Build history of the part. All positions in model axes, mm. A direction names the side the tool comes from. Round coordinates to 2 decimals unless told otherwise and drop trailing zeros. Write each loop counter-clockwise with the first axis right and the second up, starting at its lowest first coordinate (ties: lowest second). Pieces come first, ordered by that corner, then holes. Notation, with made-up numbers: (-39, 34) - (8, 34) arc R12 cw to (8, 41) - close; hole circle Ø3 at (64.25, -12). An arc over 180 degrees is marked (long way). Answer as a JSON object with one key per item and string values. Group by question number.
Item 1: Slice it at C-C, the plane z = -91. List the corners of the cut face in (x, y), then the cut area to 3 significant figures.
Item 2: Slice it at D-D, the plane x = 71. List the corners of the cut face in (y, z), then the cut area to 3 significant figures.
Item 3: Slice it at B-B, the plane y = 1.2. Give the number of separate pieces and of enclosed holes in the cut face, then the cut area to 3 significant figures.
Item 4: Which spindle directions (+Z, -Z, +X, -X, +Y, -Y) get a long thin tool onto all of the face, cutting with end or side? Do faces 4 (the cylindrical face through (-122.15, 2.46, 51.99)), 5 (the cylindrical face through (-112.97, 1.48, 47.21)). Say none if no direction does.
Item 5: Two-plate mould, pull along Z, no slides. Class faces 1 (the flat face through (43.7, 3, -46.3)), 2 (the flat face through (-30, 5, -30)), 3 (the cylindrical face through (57.85, 2.46, -58.01)): +Z half, -Z half, draft (parallel to the pull), parting line (faces both ways), or undercut.
Item 6: Flat gauge pins, fed straight in: pin 1 (6.5 mm diameter, centred on x = -113.5, z = 45, fed in from -Y); pin 2 (3 mm diameter, centred on y = 2.5, z = 99.5, fed in from -X); pin 3 (5 mm diameter, centred on x = 45, z = 45, fed in from -Y); pin 4 (3 mm diameter, centred on x = -115, z = -45, fed in from -Y). Where does each tip first touch, or does it go through?
Item 7: Slice it at A-A, the plane z = 20. List the corners of the cut face in (x, y).
Item 8: Probe line 1 (X direction, y = 3.5, z = -115); line 2 (X direction, y = 3.4, z = -45); line 3 (X direction, y = 4.45, z = -70.5). List the from-to ranges inside material, lowest first. Write a range as from..to.
from build123d import *

# Parameters (mm, degrees)
SKETCH_1_W          = 250
SKETCH_1_H          = 250
SKETCH_1_R          = 40
SKETCH_1_R_2        = 2.05
EXTRUDE_1_DEPTH     = 5
SKETCH_2_R          = 1.6
SKETCH_2_W          = 70
SKETCH_2_H          = 70
CUT_EXTRUDE_1_DEPTH = 177.847391838
FILLET_1_R          = 10
SKETCH_4_R          = 3
CUT_EXTRUDE_3_DEPTH = 3


with BuildPart() as part:
    # ｽｹｯﾁ1 → ﾎﾞｽ - 押し出し1 (new body)
    with BuildSketch(Plane(origin=(0, 0, 0), x_dir=(1, 0, 0), z_dir=(0, 1, 0))):
        Rectangle(SKETCH_1_W, SKETCH_1_H)
        with Locations(Location((0, 0, 0), (0, 0, 270))):
            Circle(SKETCH_1_R, mode=Mode.SUBTRACT)
        with Locations(Location((0, 60, 0), (0, 0, 270))):
            Circle(SKETCH_1_R_2, mode=Mode.SUBTRACT)
        with Locations(Location((60, 0, 0), (0, 0, 270))):
            Circle(SKETCH_1_R_2, mode=Mode.SUBTRACT)
        with Locations(Location((0, -60, 0), (0, 0, 270))):
            Circle(SKETCH_1_R_2, mode=Mode.SUBTRACT)
        with Locations(Location((-60, 0, 0), (0, 0, 270))):
            Circle(SKETCH_1_R_2, mode=Mode.SUBTRACT)
    extrude(amount=EXTRUDE_1_DEPTH)

    # ｽｹｯﾁ2 → ｶｯﾄ - 押し出し1 (cut, through all)
    with BuildSketch(Plane(origin=(0, 5, 0), x_dir=(1, 0, 0), z_dir=(0, 1, 0))):
        with Locations(Location((-45, 115, 0), (0, 0, 270))):
            Circle(SKETCH_2_R)
        with Locations(Location((-45, 45, 0), (0, 0, 270))):
            Circle(SKETCH_2_R)
        with Locations(Location((-115, 45, 0), (0, 0, 270))):
            Circle(SKETCH_2_R)
        with Locations(Location((115, 45, 0), (0, 0, 90))):
            Circle(SKETCH_2_R)
        with Locations(Location((45, 115, 0), (0, 0, 90))):
            Circle(SKETCH_2_R)
        with Locations(Location((45, 45, 0), (0, 0, 90))):
            Circle(SKETCH_2_R)
        with Locations(Location((-115, -45, 0), (0, 0, 90))):
            Circle(SKETCH_2_R)
        with Locations(Location((-45, -45, 0), (0, 0, 90))):
            Circle(SKETCH_2_R)
        with Locations(Location((-45, -115, 0), (0, 0, 90))):
            Circle(SKETCH_2_R)
        with Locations(Location((45, -115, 0), (0, 0, 270))):
            Circle(SKETCH_2_R)
        with Locations(Location((45, -45, 0), (0, 0, 270))):
            Circle(SKETCH_2_R)
        with Locations(Location((115, -45, 0), (0, 0, 270))):
            Circle(SKETCH_2_R)
        with Locations((-90, 90)):
            Rectangle(SKETCH_2_W, SKETCH_2_H)
        with Locations((90, 90)):
            Rectangle(SKETCH_2_W, SKETCH_2_H)
        with Locations((90, -90)):
            Rectangle(SKETCH_2_W, SKETCH_2_H)
        with Locations((-90, -90)):
            Rectangle(SKETCH_2_W, SKETCH_2_H)
    extrude(amount=-CUT_EXTRUDE_1_DEPTH, mode=Mode.SUBTRACT)

    # ﾌｨﾚｯﾄ1
    fillet_1_edges = [part.edges().sort_by_distance(p)[0] for p in [
        (-125, 2.5, -55),
        (-55, 2.5, -125),
        (-55, 2.5, -55),
        (-125, 2.5, 55),
        (-55, 2.5, 55),
        (-55, 2.5, 125),
        (55, 2.5, 125),
        (55, 2.5, 55),
        (125, 2.5, 55),
        (125, 2.5, -55),
        (55, 2.5, -55),
        (55, 2.5, -125),
    ]]
    fillet(fillet_1_edges, radius=FILLET_1_R)

    # ｽｹｯﾁ4 → ｶｯﾄ - 押し出し3 (cut)
    with BuildSketch(Plane.XZ):
        with Locations(Location((-45, 115, 0), (0, 0, 270))):
            Circle(SKETCH_4_R)
        with Locations(Location((-45, 45, 0), (0, 0, 270))):
            Circle(SKETCH_4_R)
        with Locations(Location((-115, 45, 0), (0, 0, 270))):
            Circle(SKETCH_4_R)
        with Locations(Location((115, 45, 0), (0, 0, 90))):
            Circle(SKETCH_4_R)
        with Locations(Location((45, 45, 0), (0, 0, 90))):
            Circle(SKETCH_4_R)
        with Locations(Location((45, 115, 0), (0, 0, 90))):
            Circle(SKETCH_4_R)
        with Locations(Location((45, -115, 0), (0, 0, 270))):
            Circle(SKETCH_4_R)
        with Locations(Location((45, -45, 0), (0, 0, 270))):
            Circle(SKETCH_4_R)
        with Locations(Location((115, -45, 0), (0, 0, 270))):
            Circle(SKETCH_4_R)
        with Locations(Location((-115, -45, 0), (0, 0, 90))):
            Circle(SKETCH_4_R)
        with Locations(Location((-45, -45, 0), (0, 0, 90))):
            Circle(SKETCH_4_R)
        with Locations(Location((-45, -115, 0), (0, 0, 90))):
            Circle(SKETCH_4_R)
    extrude(amount=-CUT_EXTRUDE_3_DEPTH, mode=Mode.SUBTRACT)


solid = part.part
Geometry says:
{
 "1": {"outline": "(-55, 0) - (55, 0) - (55, 5) - (-55, 5) - close", "area": "550 mm^2"},
 "2": {"outline": "(0, -55) - (5, -55) - (5, 55) - (0, 55) - close", "area": "550 mm^2"},
 "3": {"separate pieces": "1", "enclosed holes": "17", "area": "37,400 mm^2"},
 "4": {"face 4": "+Z, -X, +Y, -Y", "face 5": "-Y"},
 "5": {"face 1": "undercut", "face 2": "draft", "face 3": "-Z half"},
 "6": {"pin 1": "stops at y = 0", "pin 2": "stops at x = -55", "pin 3": "stops at y = 3", "pin 4": "passes through"},
 "7": {"outline": "(-125, 0) - (-34.64, 0) - (-34.64, 5) - (-125, 5) - close; (34.64, 0) - (125, 0) - (125, 5) - (34.64, 5) - close"},
 "8": {"line 1": "x = -55..-46.6, -43.4..43.4, 46.6..55", "line 2": "x = -125..-116.6, -113.4..-46.6, -43.4..43.4, 46.6..113.4, 116.6..125", "line 3": "x = -55..55"}
}
